Can you work these out from the model? Positions are in its coordinate system, mm. Face numbers are marked on the shaded views. Coordinates: 2 decimals unless noted, no trailing zeros. Order: outer loops, then holes, each group sorted by start corner. A loop starts at its lowest first (then second) coordinate and runs counter-clockwise, first axis right, second up. Notation, with made-up numbers: (58, 55.25) -> (100, 55.25) arc R20 cw to (100, 65.25) -> close; hole circle Ø10 at (82, 17). An arc over 180 degrees is marked (long way). Answer in a Markdown table with one row per item.
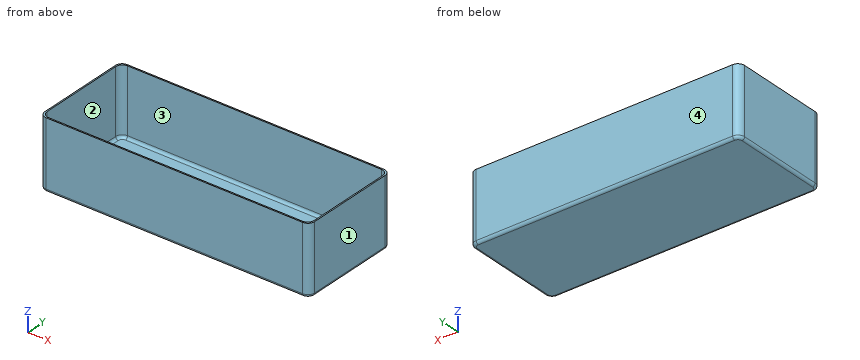
```python
from build123d import *

# Parameters (mm, degrees)
F0_W     = 202
F0_H     = 77
F1_DEPTH = 51
F2_W     = 200
F2_H     = 75
F3_DEPTH = 50
F4_R     = 5
F5_R     = 2


# Not quite as in the source:
# - a feature of the source that left no trace in its solid (it failed there, or was rolled back) is left out


with BuildPart() as f1:
    # F0 (on Top) → F1 (new body)
    with BuildSketch(Plane.XY):
        with Locations((-2.8100872189, -1.361513185)):
            Rectangle(F0_W, F0_H)
    extrude(amount=F1_DEPTH)

    # F2 (on face) → F3 (cut)
    with BuildSketch(Plane.XY.offset(51)):
        with Locations((-2.8100872189, -1.361513185)):
            Rectangle(F2_W, F2_H)
    extrude(amount=-F3_DEPTH, mode=Mode.SUBTRACT)

    # F4
    f4_edges = [f1.edges().sort_by_distance(p)[0] for p in [
        (97.189913, 36.138487, 26),
        (-102.810087, 36.138487, 26),
        (97.189913, -38.861513, 26),
        (-102.810087, -38.861513, 26),
        (98.189913, 37.138487, 25.5),
        (-103.810087, 37.138487, 25.5),
        (98.189913, -39.861513, 25.5),
        (-103.810087, -39.861513, 25.5),
    ]]
    fillet(f4_edges, radius=F4_R)

    # F5
    f5_edges = [f1.edges().sort_by_distance(p)[0] for p in [
        (97.189913, -1.361513, 1),
        (-2.810087, 36.138487, 1),
        (-2.810087, -38.861513, 1),
        (-2.810087, 37.138487, 0),
        (96.725447, 35.674021, 0),
        (-102.345621, 35.674021, 0),
        (98.189913, -1.361513, 0),
        (-103.810087, -1.361513, 0),
        (96.725447, -38.397047, 0),
        (-102.345621, -38.397047, 0),
        (-2.810087, -39.861513, 0),
        (95.725447, -37.397047, 1),
        (95.725447, 34.674021, 1),
        (-101.345621, -37.397047, 1),
        (-101.345621, 34.674021, 1),
        (-102.810087, -1.361513, 1),
    ]]
    fillet(f5_edges, radius=F5_R)


solid = f1.part
```
(1) Suppose I cut it at C-C (x = -40). Please give me the cut outline in (y, z).
Response values:
| item | result |
|---|---|
| outline | (-39.86, 2) arc R2 ccw to (-37.86, 0) -> (35.14, 0) arc R2 ccw to (37.14, 2) -> (37.14, 51) -> (36.14, 51) -> (36.14, 3) arc R2 cw to (34.14, 1) -> (-36.86, 1) arc R2 cw to (-38.86, 3) -> (-38.86, 51) -> (-39.86, 51) -> close |
(2) Suppose I cut it at B-B (y = -11.5). Please give me the cut outline in (x, z), and give its area (3 significant figures).
Response values:
| item | result |
|---|---|
| outline | (-103.81, 2) arc R2 ccw to (-101.81, 0) -> (96.19, 0) arc R2 ccw to (98.19, 2) -> (98.19, 51) -> (97.19, 51) -> (97.19, 3) arc R2 cw to (95.19, 1) -> (-100.81, 1) arc R2 cw to (-102.81, 3) -> (-102.81, 51) -> (-103.81, 51) -> close |
| area | 302 mm2 |
(3) Will this pin go through, and if not, where does the flat tip stop? pin 1 Ø5 at (x, y) = (64, 21.5) entering from +Z.
Response values:
| item | result |
|---|---|
| pin 1 | z = 1 |
(4) I need wall thicknesses on line 1 (Y direction, x = -84.5, z = 20); line 2 (X direction, y = -16, z = 25); line 3 (Z direction, x = 32.5, y = -32). Which ranges of each line are inside material? Lowest first, please. Write a range as [from, to].
Response values:
| item | result |
|---|---|
| line 1 | [-39.86, -38.86], [36.14, 37.14] |
| line 2 | [-103.81, -102.81], [97.19, 98.19] |
| line 3 | [0, 1] |
(5) We'd pull the mould along X, two halves only. Please class the marked faces 1, 2, 3 and 4: +X half, -X half, draft (parallel to the pull), parting line (faces both ways), or undercut.
Response values:
| item | result |
|---|---|
| face 1 | +X half |
| face 2 | undercut |
| face 3 | undercut |
| face 4 | draft |
(6) Suppose I cut it at A-A (z = 23). Please give me the cut outline in (x, y).
Response values:
| item | result |
|---|---|
| outline | (-103.81, -34.86) arc R5 ccw to (-98.81, -39.86) -> (93.19, -39.86) arc R5 ccw to (98.19, -34.86) -> (98.19, 32.14) arc R5 ccw to (93.19, 37.14) -> (-98.81, 37.14) arc R5 ccw to (-103.81, 32.14) -> close; hole (-102.81, -33.86) arc R5 ccw to (-97.81, -38.86) -> (92.19, -38.86) arc R5 ccw to (97.19, -33.86) -> (97.19, 31.14) arc R5 ccw to (92.19, 36.14) -> (-97.81, 36.14) arc R5 ccw to (-102.81, 31.14) -> close |
